Design review of the part built by this model. Coordinates are the model's own, in mm. Coordinates: 2 decimals unless noted, no trailing zeros. Loops run counter-clockwise (first coordinate to the right, second up) from the corner with the lowest first, then second, coordinate; pieces in that order, holes last. Notation, with made-up numbers: M 86.5,5.5 L 144.5,5.5 A36 cw 144.5,44.5 Z; hole C -29.75,47.25 d11. An arc over 180 degrees is marked long. Answer as a JSON object with one key per item and string values. Group by question number.
1. Insertion check: pin 1 (0.9 mm diameter, centred on y = 1.5, z = 26.5, fed in from +X); pin 2 (0.9 mm diameter, centred on x = -28, y = 1, fed in from +Z); pin 3 (0.9 mm diameter, centred on y = 1, z = 31.5, fed in from -X); pin 4 (2.5 mm diameter, centred on x = -40, z = 10, fed in from -Y). Each pin has a flat end and moves straight along its axis. Give the tip position at first contact, or say it passes through.
2. Consider section A-A (z = 22). State the section outline as (x, y) points.
3. Consider section B-B (y = 1.05). Count the separate pieces of the cut face and the enclosed holes in it, then the cut area to 3 significant figures.
4. To check wall thickness, follow probe 1 along Z at (x, y) = (-40, 0.65); probe 2 along X at (y, z) = (1.45, 10); probe 3 along X at (y, z) = (2.2, -29.5). State the ranges of each line that lie inside material, in increasing order.
5. Consider section C-C (x = -27.5). State the section outline as (y, z) points.
from build123d import *

# Parameters (mm, degrees)
SKETCH_1_R          = 1.5
EXTRUDE_1_DEPTH     = 5
CUT_EXTRUDE_1_DEPTH = 10
SKETCH_3_W          = 97.68283175
SKETCH_3_H          = 2
CUT_EXTRUDE_2_DEPTH = 94


with BuildPart() as part:
    # 草图1 → 凸台-拉伸1 (new body)
    with BuildSketch(Plane(origin=(0, 0, 0), x_dir=(1, 0, 0), z_dir=(0, 1, 0))):
        with BuildLine():
            Line((14, -40), (14, -18))
            ThreePointArc((14, -18), (15.171572875, -15.171572875), (18, -14))
            Line((18, -14), (40, -14))
            ThreePointArc((40, -14), (42.828427125, -12.828427125), (44, -10))
            Line((44, -10), (44, 10))
            ThreePointArc((44, 10), (42.828427125, 12.828427125), (40, 14))
            Line((40, 14), (18, 14))
            ThreePointArc((18, 14), (15.171572875, 15.171572875), (14, 18))
            Line((14, 18), (14, 40))
            ThreePointArc((14, 40), (12.828427125, 42.828427125), (10, 44))
            Line((10, 44), (-10, 44))
            ThreePointArc((-10, 44), (-12.828427125, 42.828427125), (-14, 40))
            Line((-14, 40), (-14, 18))
            ThreePointArc((-14, 18), (-15.171572875, 15.171572875), (-18, 14))
            Line((-18, 14), (-40, 14))
            ThreePointArc((-40, 14), (-42.828427125, 12.828427125), (-44, 10))
            Line((-44, 10), (-44, -10))
            ThreePointArc((-44, -10), (-42.828427125, -12.828427125), (-40, -14))
            Line((-40, -14), (-18, -14))
            ThreePointArc((-18, -14), (-15.171572875, -15.171572875), (-14, -18))
            Line((-14, -18), (-14, -40))
            ThreePointArc((-14, -40), (-12.828427125, -42.828427125), (-10, -44))
            Line((-10, -44), (10, -44))
            ThreePointArc((10, -44), (12.828427125, -42.828427125), (14, -40))
        make_face()
        with Locations(Location((40, 10, 0), (0, 0, 270))):
            Circle(SKETCH_1_R, mode=Mode.SUBTRACT)
        with Locations(Location((40, -10, 0), (0, 0, 270))):
            Circle(SKETCH_1_R, mode=Mode.SUBTRACT)
        with Locations(Location((-40, 10, 0), (0, 0, 270))):
            Circle(SKETCH_1_R, mode=Mode.SUBTRACT)
        with Locations(Location((-40, -10, 0), (0, 0, 270))):
            Circle(SKETCH_1_R, mode=Mode.SUBTRACT)
        with BuildLine():
            ThreePointArc((-2.7, 30), (0, 27.3), (2.7, 30))
            Line((2.7, 30), (2.7, 35))
            ThreePointArc((2.7, 35), (0, 37.7), (-2.7, 35))
            Line((-2.7, 35), (-2.7, 30))
        make_face(mode=Mode.SUBTRACT)
        with BuildLine():
            ThreePointArc((2.7, -30), (0, -27.3), (-2.7, -30))
            Line((-2.7, -30), (-2.7, -35))
            ThreePointArc((-2.7, -35), (0, -37.7), (2.7, -35))
            Line((2.7, -35), (2.7, -30))
        make_face(mode=Mode.SUBTRACT)
    extrude(amount=EXTRUDE_1_DEPTH)

    # 草图2 → 切除-拉伸1 (cut)
    with BuildSketch(Plane.XZ):
        with BuildLine():
            Line((-2.7, -21), (-2.7, -30))
            ThreePointArc((-2.7, -30), (0, -27.3), (2.7, -30))
            Line((2.7, -30), (2.7, -21))
            ThreePointArc((2.7, -21), (0, -18.3), (-2.7, -21))
        make_face()
        with BuildLine():
            ThreePointArc((2.7, 30), (0, 27.3), (-2.7, 30))
            Line((-2.7, 30), (-2.7, 21))
            ThreePointArc((-2.7, 21), (0, 18.3), (2.7, 21))
            Line((2.7, 21), (2.7, 30))
        make_face()
        with BuildLine():
            ThreePointArc((-2.7, -30), (0, -27.3), (2.7, -30))
            Line((2.7, -30), (2.7, -35))
            ThreePointArc((2.7, -35), (0, -37.7), (-2.7, -35))
            Line((-2.7, -35), (-2.7, -30))
        make_face()
        with BuildLine():
            ThreePointArc((2.7, 30), (0, 27.3), (-2.7, 30))
            Line((-2.7, 30), (-2.7, 35))
            ThreePointArc((-2.7, 35), (0, 37.7), (2.7, 35))
            Line((2.7, 35), (2.7, 30))
        make_face()
    extrude(amount=-CUT_EXTRUDE_1_DEPTH, mode=Mode.SUBTRACT)

    # 草图3 → 切除-拉伸2 (cut)
    with BuildSketch(Plane.XY.offset(44)):
        with Locations((4.841415875, 4)):
            Rectangle(SKETCH_3_W, SKETCH_3_H)
    extrude(amount=-CUT_EXTRUDE_2_DEPTH, mode=Mode.SUBTRACT)


solid = part.part
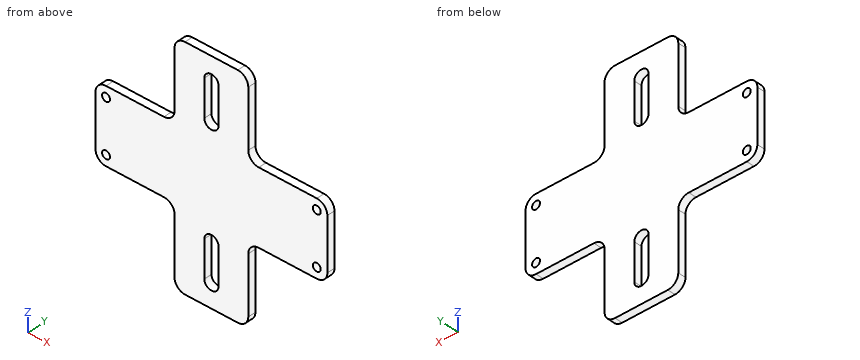
Findings below:
{
 "1": {"pin 1": "stops at x = 14", "pin 2": "stops at z = 14", "pin 3": "stops at x = -14", "pin 4": "passes through"},
 "2": {"outline": "M -14,0 L -2.7,0 L -2.7,3 L -14,3 Z; M 2.7,0 L 14,0 L 14,3 L 2.7,3 Z"},
 "3": {"separate pieces": "1", "enclosed holes": "6", "area": "3,900 mm^2"},
 "4": {"probe 1": "z = -14 to -11.5, -8.5 to 8.5, 11.5 to 14", "probe 2": "x = -44 to -41.5, -38.5 to 38.5, 41.5 to 44", "probe 3": "x = -14 to -2.7, 2.7 to 14"},
 "5": {"outline": "M 0,-14 L 3,-14 L 3,14 L 0,14 Z"}
}
